```python
from build123d import *

# Parameters (mm, degrees)
F0_R     = 2.0701
F1_DEPTH = 73.9775
F3_DEPTH = 73.9648
F5_DEPTH = 33.1978
F6_DEPTH = 38.1127


with BuildPart() as f1:
    # F0 (on Right) → F1 (new body, symmetric)
    with BuildSketch(Plane.YZ):
        Circle(F0_R)
    extrude(amount=F1_DEPTH, both=True)

    # F2 (on Right) → F3 (join)
    with BuildSketch(Plane.YZ):
        with BuildLine():
            ThreePointArc((-2.3136596952, 1.2537271952), (-0.6466957718, -2.5508111737), (2.6315115552, 0))
            ThreePointArc((2.6315115552, 0), (2.5508111737, 0.6466957718), (2.3136596952, 1.2537271952))
            ThreePointArc((2.3136596952, 1.2537271952), (0, 2.6315115552), (-2.3136596952, 1.2537271952))
        make_face()
        with BuildLine():
            ThreePointArc((-2.3136596952, 1.2537271952), (0, 2.6315115552), (2.3136596952, 1.2537271952))
            Line((2.3136596952, 1.2537271952), (0.8742138073, 5.0605748032))
            ThreePointArc((0.8742138073, 5.0605748032), (0.9193959303, 4.8980330409), (0.9346220049, 4.7300169244))
            ThreePointArc((0.9346220049, 4.7300169244), (-0.1680161165, 3.8106209941), (-0.8742138073, 5.0605748032))
            Line((-0.8742138073, 5.0605748032), (-2.3136596952, 1.2537271952))
        make_face()
        with BuildLine():
            ThreePointArc((0.9346220049, 4.7300169244), (0.9193959303, 4.8980330409), (0.8742138073, 5.0605748032))
            ThreePointArc((0.8742138073, 5.0605748032), (0, 5.6646389293), (-0.8742138073, 5.0605748032))
            ThreePointArc((-0.8742138073, 5.0605748032), (-0.1680161165, 3.8106209941), (0.9346220049, 4.7300169244))
        make_face()
    extrude(amount=-F3_DEPTH)

    # F5 (cut): a face of the model
    f5_faces = [f1.faces().sort_by_distance(p)[0] for p in [
        (-73.9648, 0, -2.5332641506),
    ]]
    extrude(f5_faces, amount=-F5_DEPTH, mode=Mode.SUBTRACT)

    # F6 (cut): a face of the model
    f6_faces = [f1.faces().sort_by_distance(p)[0] for p in [
        (0, 0, -2.5332641506),
    ]]
    extrude(f6_faces, amount=-F6_DEPTH, mode=Mode.SUBTRACT)


solid = f1.part
```
CAD build for the part. Positions are in the model's coordinates, mm. A direction names the side the tool comes from. Coordinates: 2 decimals unless noted, no trailing zeros. Order: outer loops, then holes, each group sorted by start corner. A loop starts at its lowest first (then second) coordinate and runs counter-clockwise, first axis right, second up.
(1) Pin check, flat tips, straight feed: pin 1 Ø1 at (x, y) = (34, 1.5) entering from -Z; pin 2 Ø4 at (x, z) = (32.5, 1) entering from -Y; pin 3 Ø3 at (x, y) = (17.5, 0) entering from +Z. Stop position of each tip, or through.
Solution:
pin 1: stops at z = -1.81
pin 2: stops at y = -2.07
pin 3: stops at z = 2.07
(2) Saw through at B-B, the plane x = 34. Write the cut outline in (y, z), and give its area (3 significant figures).
Solution:
outline: circle Ø4.14 at (0, 0)
area: 13.5 mm2
(3) Saw through at A-A, the plane y = 0. Write the cut outline in (x, z), and give its area (3 significant figures).
Solution:
outline: (-73.98, -2.07) - (-40.77, -2.07) - (-40.77, -2.63) - (-38.11, -2.63) - (-38.11, -2.07) - (73.98, -2.07) - (73.98, 2.07) - (-38.11, 2.07) - (-38.11, 5.66) - (-40.77, 5.66) - (-40.77, 2.07) - (-73.98, 2.07) - close
area: 624 mm2
(4) Which spindle directions (+Z, -Z, +X, -X, +Y, -Y) get a long thin tool onto all of the face, cutting with end or side? Do faces 1 (the face through (-38.113, 0, 2.5)), 2 (the face through (-40.767, 0, 2.5)), 3 (the face through (73.978, 0, 0)). Say none if no direction does.
Solution:
face 1: +X
face 2: -X
face 3: +Z, -Z, +X, +Y, -Y
(5) Drill centre lines: L1, parallel to X at y = -1.95, z = 1.25; L2, parallel to Z at x = 3.5, y = -1.2; L3, parallel to Y at x = 7, z = 1.5. Where is each one in solid material? Low to high.
Solution:
L1: x = -40.77 to -38.11
L2: z = -1.69 to 1.69
L3: y = -1.43 to 1.43
